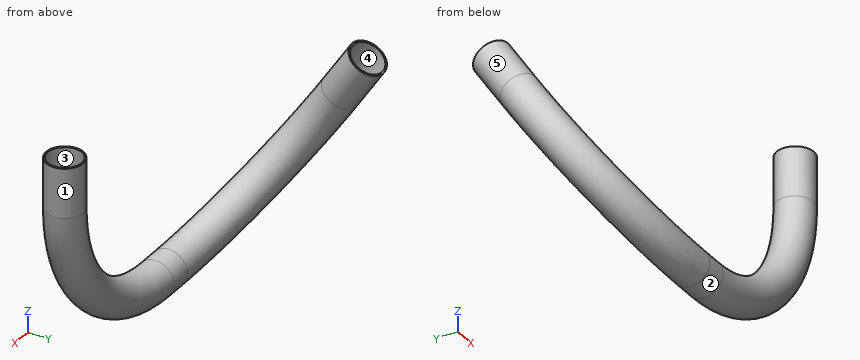
```python
from build123d import *

# Parameters (mm, degrees)
SKETCH5_R            = 19.05
SKETCH5_R_2          = 17.399
SWEEP2_START         = -50.8000001
SWEEP2_OUTLINE_R     = 19.05
SWEEP2_OUTLINE_R_2   = 17.399
SWEEP2_DEPTH         = 50.8000001
SWEEP2_2_OUTLINE_R   = 19.05
SWEEP2_2_OUTLINE_R_2 = 17.399
SWEEP2_2_ANGLE       = 90


with BuildPart() as part:
    # Sweep1: sweep along a path in Sketch4
    with BuildLine(Plane(origin=(0, 92.816218496, -60.275557063), x_dir=(1, 0, 0), z_dir=(0, 0.8386705679454234, -0.5446390350150281))) as sweep1_path:
        Line((174.625, 170.417859407), (152.4, 170.417859407))
        ThreePointArc((152.4, 170.417859407), (44.636926547, 125.780932859), (0, 18.017859407))
        Line((0, 18.017859407), (0, -32.782140593))
    # Sketch5 → Sweep1 (sweep)
    with BuildSketch(Plane(origin=(327.025, 110.670651915, -32.782140593), x_dir=(1, 0, 0), z_dir=(0, 0.5446390350150281, 0.8386705679454234))):
        with Locations((-327.025, 0)):
            Circle(SKETCH5_R)
        with Locations((-327.025, 0)):
            Circle(SKETCH5_R_2, mode=Mode.SUBTRACT)
    sweep(path=sweep1_path.line)



with BuildPart() as body_2:
    # Sweep2: read off the stored shape, not the designer's step
    # Sweep2 outline → Sweep2 (new body)
    with BuildSketch(Plane.XY.offset(SWEEP2_START)):
        with Locations((327.025, 0)):
            Circle(SWEEP2_OUTLINE_R)
        with Locations((327.025, 0)):
            Circle(SWEEP2_OUTLINE_R_2, mode=Mode.SUBTRACT)
    extrude(amount=SWEEP2_DEPTH)


with BuildPart() as part_1:
    add(part.part)

    add(body_2.part)  # Sweep2 2 merges body 2
    # Sweep2 2 outline → Sweep2 2 (revolve)
    with BuildSketch(Plane(origin=(174.625, 0, -50.8), x_dir=(1, 0, 0), z_dir=(0, 0, 1))):
        with Locations((152.4, 0)):
            Circle(SWEEP2_2_OUTLINE_R)
        with Locations((152.4, 0)):
            Circle(SWEEP2_2_OUTLINE_R_2, mode=Mode.SUBTRACT)
    revolve(axis=Axis((174.625, 0, -50.8), (0, 1, 0)), revolution_arc=SWEEP2_2_ANGLE)


solid = part_1.part
```
Model file for the job. Use its own axes, mm. Face numbers are marked on the shaded views. A direction names the side the tool comes from. Coordinates: 2 decimals unless noted, no trailing zeros. One line per item, written item: value. Start each with the question number.
1. Mould opens along X. For the marked faces 3, 4 and 5 say: released by +X, released by -X, zero draft, split by the parting line, or undercut.
2. Flat gauge pins, fed straight in: pin 1 (8 mm diameter, centred on y = 39.5, z = -114.5, fed in from -X); pin 2 (2 mm diameter, centred on y = 88.5, z = -54.5, fed in from +X); pin 3 (1.5 mm diameter, centred on x = 309, z = -107, fed in from +Y). Where does each tip first touch, or does it go through?
3. Probe line 1 (Y direction, x = 209, z = -198.5); line 2 (Z direction, x = 167.5, y = 0); line 3 (X direction, y = 11, z = -68). List the from-to ranges inside material, lowest first. Write a range as from..to.
4. Tool access for the marked faces 1 and 2: list every direction of +Z, -Z, +X, -X, +Y, -Y with a clear straight run to the whole face (end or side of a thin tool).
5. Slice it at A-A (z = -91). Count the separate pieces of the cut face and the enclosed holes in it, plus the area to 3 significant figures.
Answers below:
1. face 3: undercut
1. face 4: undercut
1. face 5: split by the parting line
2. pin 1: stops at x = -5.93
2. pin 2: stops at x = 18.16
2. pin 3: stops at y = 18.08
3. line 1: y = -19.04..-17.38, 17.38..19.04
3. line 2: z = -222.25..-220.6, -185.8..-184.15
3. line 3: x = 310.39..312.48, 339.61..341.7
4. face 1: +Z
4. face 2: none
5. separate pieces: 2
5. enclosed holes: 2
5. area: 424 mm^2
